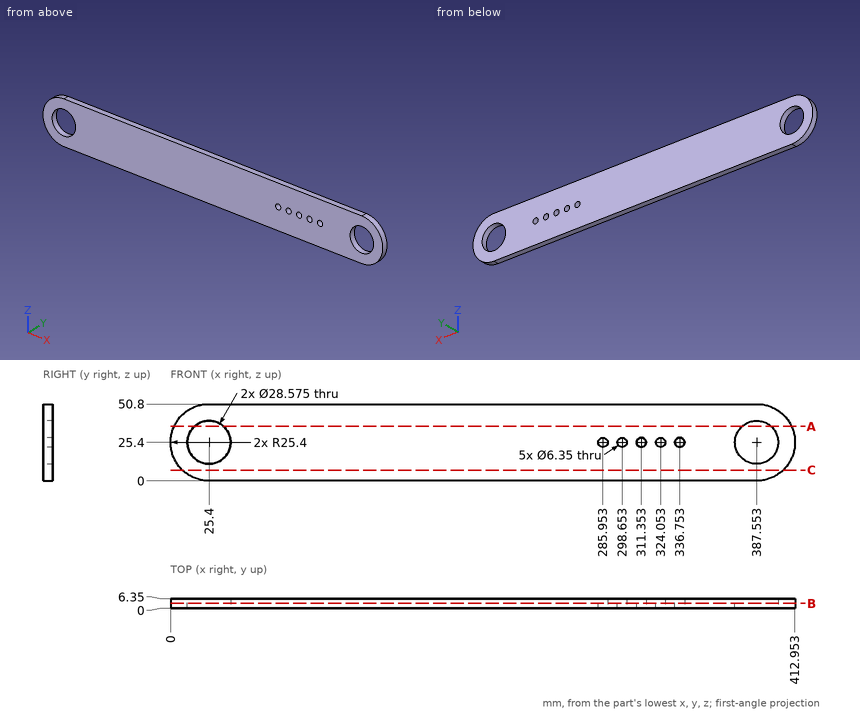
Source: three-view drawing plus pictorial views. Frame: mm from the lowest corner of the part. Coordinates: 2 decimals unless noted, no trailing zeros. Loops run counter-clockwise (first coordinate to the right, second up) from the corner with the lowest first, then second, coordinate; pieces in that order, holes last. Notation, with made-up numbers: (20, -10) - (52, -10) arc R15 cw to (52, 3) - close; hole circle Ø8 at (34.5, 2.25). An arc over 180 degrees is marked (long way). Answer in a Markdown table with one row per item. Add a question column.
Item 1: Section query A-A on z = 36. Return the cut outline in (x, y).
Item 2: Section query B-B on y = 3.25. State how many separate pieces and enclosed holes the cut face has, then the cut area to 3 significant figures.
Item 3: Contact query for a flat-ended pin moving along its axis: P1, Ø4, axis at x = 336.75, z = 25.4, coming from the -Y side. Output: stop coordinate, or through.
Item 4: Line query: line 1 along Z through (x, y) = (323.5, 5.75); line 2 along X through (y, z) = (5.75, 13.5) (1 decimal); line 3 along X through (y, z) = (1.5, 22) (1 decimal). Output: solid intervals per line, ascending. Write a range as [from, to].
Item 5: Section query C-C on z = 7. Return the cut outline in (x, y).
Recorded:
| question | item | result |
|---|---|---|
| 1 | outline | (2.32, 0) - (15.82, 0) - (15.82, 6.35) - (2.32, 6.35) - close; (34.98, 0) - (377.97, 0) - (377.97, 6.35) - (34.98, 6.35) - close; (397.13, 0) - (410.64, 0) - (410.64, 6.35) - (397.13, 6.35) - close |
| 2 | separate pieces | 1 |
| 2 | enclosed holes | 7 |
| 2 | area | 19,000 mm^2 |
| 3 | P1 | through |
| 4 | line 1 | [0, 22.27], [28.53, 50.8] |
| 4 | line 2 | [3, 17.5], [33.3, 379.6], [395.5, 410] |
| 4 | line 3 | [0.2, 11.5], [39.3, 373.7], [401.4, 412.7] |
| 5 | outline | (7.89, 0) - (405.06, 0) - (405.06, 6.35) - (7.89, 6.35) - close |
